Job drawing, mm, ordinate dimensions from the low corner. One solid piece. A direction names the side the tool comes from. Give positions to 0.01 mm unless a question says otherwise; leave off trailing zeros. Order: outer loops, then holes, each group sorted by start corner. A loop starts at its lowest first (then second) coordinate and runs counter-clockwise, first axis right, second up. Notation, with made-up numbers: (-21, 35.5) - (35, 35.5) arc R32 cw to (35, 67.5) - close; hole circle Ø11 at (11, 39.5). An arc over 180 degrees is marked (long way). Use one line per item in the form item = value. Start each with the question number.
1. Tool access for the marked faces 1 and 2: list every direction of +Z, -Z, +X, -X, +Y, -Y with a clear straight run to the whole face (end or side of a thin tool).
2. Drill centre lines: line 1 (Y direction, x = 9.5, z = 24.75); line 2 (Z direction, x = 5.75, y = 17.5); line 3 (X direction, y = 11.25, z = 17.5). Where is each one in solid material? Low to high.
3. Band-saw the part on C-C, the plane y = 3.25. List the corners of the cut face in (x, z), plus the area to 3 significant figures.
4. Pull direction Y, two halves, no side cores. Call the marked faces 3, 4 and 5: +Y half, -Y half, draft (parallel to the pull), parting line (faces both ways), or undercut.
5. Band-saw the part on B-B, the plane x = 9. List the corners of the cut face in (y, z), plus the area to 3 significant figures.
6. Band-saw the part on A-A, the plane z = 21.5. List the corners of the cut face in (x, y) (3 decimals), plus the area to 3 significant figures.
7. Pin check, flat tips, straight feed: P1, Ø8, axis at x = 8.5, z = 13.5, coming from the +Y side (3 decimals); P2, Ø4, axis at x = 9.525, z = 22, coming from the -Y side (3 decimals); P3, Ø6, axis at y = 6, z = 7.5, coming from the +X side. Stop position of each tip, or through.
8. Band-saw the part on D-D, the plane z = 4.75. List the corners of the cut face in (x, y) (3 decimals), plus the area to 3 significant figures.
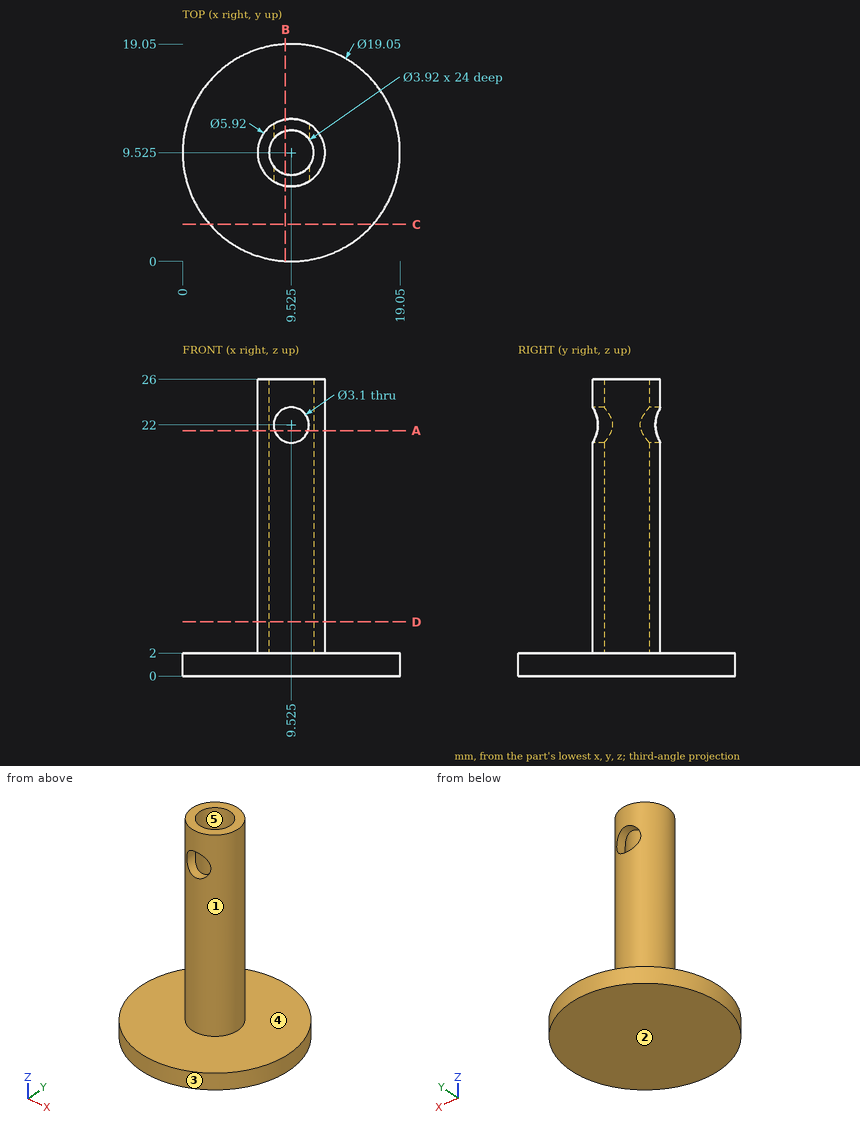
From the geometry:
q1.face_1 = +Z
q1.face_2 = -Z, +X, -X, +Y, -Y
q2.line_1 = 6.57 to 7.57, 11.48 to 12.48
q2.line_2 = 0 to 2
q2.line_3 = 7.12 to 8.59, 10.46 to 11.93
q3.outline = (2.36, 0) - (16.69, 0) - (16.69, 2) - (2.36, 2) - close
q3.area = 28.7 mm²
q4.face_3 = parting line
q4.face_4 = draft
q4.face_5 = undercut
q5.outline = (0.01, 0) - (19.04, 0) - (19.04, 2) - (12.44, 2) - (12.44, 20.54) - (11.41, 20.54) - (11.41, 2) - (7.64, 2) - (7.64, 20.54) - (6.61, 20.54) - (6.61, 2) - (0.01, 2) - close; (6.61, 23.46) - (7.64, 23.46) - (7.64, 26) - (6.61, 26) - close; (11.41, 23.46) - (12.44, 23.46) - (12.44, 26) - (11.41, 26) - close
q5.area = 81.2 mm²
q6.outline = (8.058, 6.954) - (8.058, 8.225) arc R1.96 cw to (8.058, 10.825) - (8.058, 12.096) arc R2.96 ccw to start; (10.992, 6.954) arc R2.96 ccw to (10.992, 12.096) - (10.992, 10.825) arc R1.96 cw to (10.992, 8.225) - close
q6.area = 9.14 mm²
q7.P1 = 12.485
q7.P2 = 6.565
q7.P3 = 12.44
q8.outline = circle Ø5.92 at (9.525, 9.525); hole circle Ø3.92 at (9.525, 9.525)
q8.area = 15.5 mm²
